For this review, take the finished solid that the model builds, in its own axes (mm). A direction names the side the tool comes from. Round coordinates to 2 decimals unless told otherwise and drop trailing zeros. Write each loop counter-clockwise with the first axis right and the second up, starting at its lowest first coordinate (ties: lowest second). Pieces come first, ordered by that corner, then holes. Notation, with made-up numbers: (-15, 31.5) -> (29, 31.5) arc R21 cw to (29, 49.5) -> close; hole circle Ø5 at (89, 43.25). An arc over 180 degrees is marked (long way). Answer in a Markdown table with one row per item.
from build123d import *

# Parameters (mm, degrees)
EXTRUDE7_DEPTH = 76.2
EXTRUDE8_REACH = 138.595
SKETCH17_R     = 5.268795673
FILLET1_R      = 4.7752


with BuildPart() as part:
    # Sketch16 → Extrude7 (new body)
    with BuildSketch(Plane(origin=(0, 0, 0), x_dir=(0, 0, -1), z_dir=(1, 0, 0))):
        Polygon((0, 0), (107.851907976, 0), (107.851907976, 34.925), (75.287725604, 34.925), (63.942784648, 9.525), (0, 9.525), align=None)
    extrude(amount=EXTRUDE7_DEPTH)

    # Extrude8: up to this plane
    extrude8_end = Plane(origin=(76.2, 34.925, -75.287725604), z_dir=(0, -0.4078203414676676, -0.9130621934376623))
    # Sketch17 → Extrude8 (add, up to the surface)
    with BuildSketch(Plane.XY, mode=Mode.PRIVATE) as extrude8_sk1:
        with BuildLine():
            Line((39.116, 9.525), (37.084, 9.525))
            Line((37.084, 9.525), (37.084, 12.7))
            Line((37.084, 12.7), (37.084, 12.777118098))
            ThreePointArc((37.084, 12.777118098), (38.1, 26.162510517), (39.116, 12.777118098))
            Line((39.116, 12.777118098), (39.116, 12.7))
            Line((39.116, 12.7), (39.116, 9.525))
        make_face()
        with Locations((38.1, 19.431255259)):
            Circle(SKETCH17_R, mode=Mode.SUBTRACT)
    extrude8_tool1 = split(extrude(extrude8_sk1.sketch, amount=-EXTRUDE8_REACH, mode=Mode.PRIVATE), bisect_by=extrude8_end, keep=Keep.BOTH, mode=Mode.PRIVATE)
    add(extrude8_tool1.solids().sort_by_distance((38.1, 9.73902, 0))[0])

    # Fillet1
    fillet1_edges = [part.edges().sort_by_distance(p)[0] for p in [
        (57.658, 9.525, -63.942784648),
        (18.542, 9.525, -63.942784648),
    ]]
    fillet(fillet1_edges, radius=FILLET1_R)


solid = part.part
1) For faces 5 (the flat face through (37.084, 11, -32)), 6 (the flat face through (39.116, 11, -32)), 7 (the cylindrical face through (37.818, 26.157, -35.313)), 8 (the flat face through (76.2, 14, -77)), 9 (the flat face through (38, 17, -107.852)), list the 3-axis set-ups (+Z, -Z, +X, -X, +Y, -Y) from which the entire face can be reached by the end or side of a thin tool; tool diameter is ignored.
Solved:
| item | result |
|---|---|
| face 5 | +Z, -X |
| face 6 | +Z, +X |
| face 7 | +Z |
| face 8 | +Z, -Z, +X, +Y, -Y |
| face 9 | -Z, +X, -X, +Y, -Y |
2) Consider section B-B on z = -52. State the section outline as (x, y) points (3 decimals).
Solved:
| item | result |
|---|---|
| outline | (0, 0) -> (76.2, 0) -> (76.2, 9.525) -> (39.116, 9.525) -> (39.116, 12.777) arc R6.731 ccw (long way) to (37.084, 12.777) -> (37.084, 9.525) -> (0, 9.525) -> close; hole circle Ø10.538 at (38.1, 19.431) |
3) Mouldability with a two-part tool opening along X and no side actions: class faces 1 (the flat face through (38, 0, -53)), 2 (the cylindrical face through (37.414, 24.655, -34.893)), 3 (the flat face through (0, 14, -77)), 4 (the flat face through (38, 19.5, -68.4)) as pulls with the +X half, pulls with the -X half, needs draft (parallel to the pull), parting line crosses it, or undercut.
Solved:
| item | result |
|---|---|
| face 1 | needs draft |
| face 2 | undercut |
| face 3 | pulls with the -X half |
| face 4 | undercut |
4) Consider section C-C on y = 16.5. State the section outline as (x, z) points.
Solved:
| item | result |
|---|---|
| outline | (0, -107.85) -> (76.2, -107.85) -> (76.2, -67.06) -> (44.16, -67.06) -> (44.16, 0) -> (42.48, 0) -> (42.48, -67.06) -> (33.72, -67.06) -> (33.72, 0) -> (32.04, 0) -> (32.04, -67.06) -> (0, -67.06) -> close |
5) Consider section D-D on y = 33.5. State the section outline as (x, z) points.
Solved:
| item | result |
|---|---|
| outline | (0, -107.85) -> (76.2, -107.85) -> (76.2, -74.65) -> (0, -74.65) -> close |
6) Consider section A-A on x = 11.5. State the section outline as (y, z) points (3 decimals), then the cut area to 3 significant figures.
Solved:
| item | result |
|---|---|
| outline | (0, -107.852) -> (34.925, -107.852) -> (34.925, -75.288) -> (12.353, -65.206) arc R4.775 cw to (9.525, -60.846) -> (9.525, 0) -> (0, 0) -> close |
| area | 2,000 mm² |
7) For line 1 (Y direction, x = 38.1, z = -13.5); line 2 (Y direction, x = 27.5, z = -46.5) (3 decimals); line 3 (X direction, y = 16, z = -32), list the stretches that pass through material, from the lowest coordinate up. Write a range as [from, to].
Solved:
| item | result |
|---|---|
| line 1 | [0, 14.16], [24.7, 26.16] |
| line 2 | [0, 9.525] |
| line 3 | [32.31, 34.1], [42.1, 43.89] |
8) Clearance check with flat-ended pins moving along their axes: pin 1 Ø11 at (x, z) = (11.5, -42) entering from +Y (3 decimals); pin 2 Ø1.6 at (y, z) = (11.5, -29.5) entering from -X; pin 3 Ø5 at (y, z) = (27, -51) entering from +X. State where each tip first meets the part, or that it passes through.
Solved:
| item | result |
|---|---|
| pin 1 | y = 9.525 |
| pin 2 | x = 37.08 |
| pin 3 | x = 42.53 |
